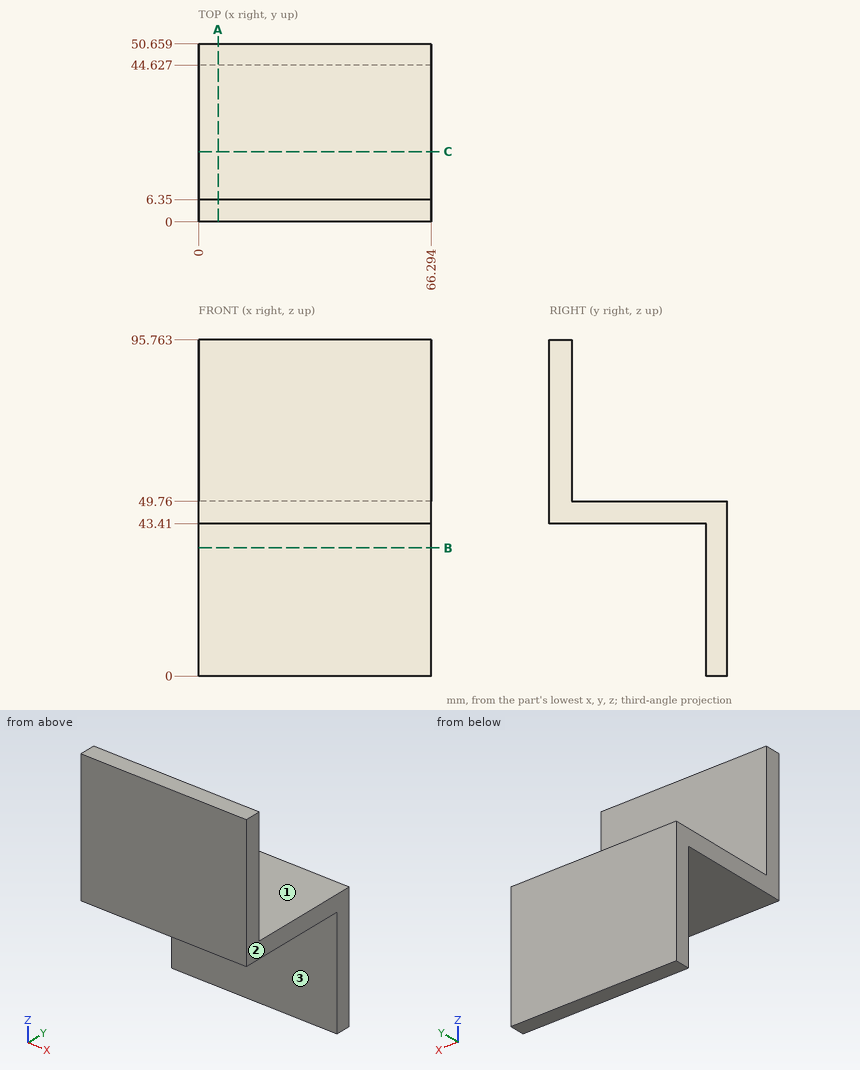
Geometry check sheet. Reference: drawing and pictorial views, mm from the part's lowest x, y, z. A direction names the side the tool comes from. Round coordinates to 2 decimals unless told otherwise and drop trailing zeros. Loops run counter-clockwise (first coordinate to the right, second up) from the corner with the lowest first, then second, coordinate; pieces in that order, holes last. Notation, with made-up numbers: (76.5, -36.75) - (105.5, -36.75) arc R13 ccw to (105.5, -11.75) - close; hole circle Ø5 at (55.25, -37). An arc over 180 degrees is marked (long way). Write item = value, one per line. Start each with the question number.
Q1. Section check B-B (z = 36.5). Record the boundary of the cut face in (x, y), plus the area to 3 significant figures.
Q2. Section check C-C (y = 20). Record the boundary of the cut face in (x, z).
Q3. Section check A-A (x = 5.5). Record the boundary of the cut face in (y, z).
Q4. Thickness scan on L1, parallel to Y at x = 50.5, z = 28; L2, parallel to Z at x = 47, y = 6.5; L3, parallel to Y at x = 3, z = 69.5. Record the ranges inside material, lowest first.
Q5. Access from +Z, -Z, +X, -X, +Y, -Y to the whole of each face (thin tool, end or side, straight path). Record for the marked faces 1, 2 and 3.
Q6. Depth check by flat-ended pin: P1, Ø8, axis at x = 36.5, y = 45, coming from the +Z side; P2, Ø14, axis at x = 20.5, z = 82.5, coming from the +Y side; P3, Ø21.5, axis at x = 34, z = 18, coming from the -Y side. Enter the tip coordinate at first touch or a pass-through.
Derived:
q1.outline = (0, 44.63) - (66.29, 44.63) - (66.29, 50.66) - (0, 50.66) - close
q1.area = 400 mm^2
q2.outline = (0, 43.41) - (66.29, 43.41) - (66.29, 49.76) - (0, 49.76) - close
q3.outline = (0, 43.41) - (44.63, 43.41) - (44.63, 0) - (50.66, 0) - (50.66, 49.76) - (6.35, 49.76) - (6.35, 95.76) - (0, 95.76) - close
q4.L1 = 44.63 to 50.66
q4.L2 = 43.41 to 49.76
q4.L3 = 0 to 6.35
q5.face_1 = +Z, +X, -X, +Y
q5.face_2 = +Z, -Z, +X, +Y, -Y
q5.face_3 = -Z, +X, -X, -Y
q6.P1 = 49.76
q6.P2 = 6.35
q6.P3 = 44.63
